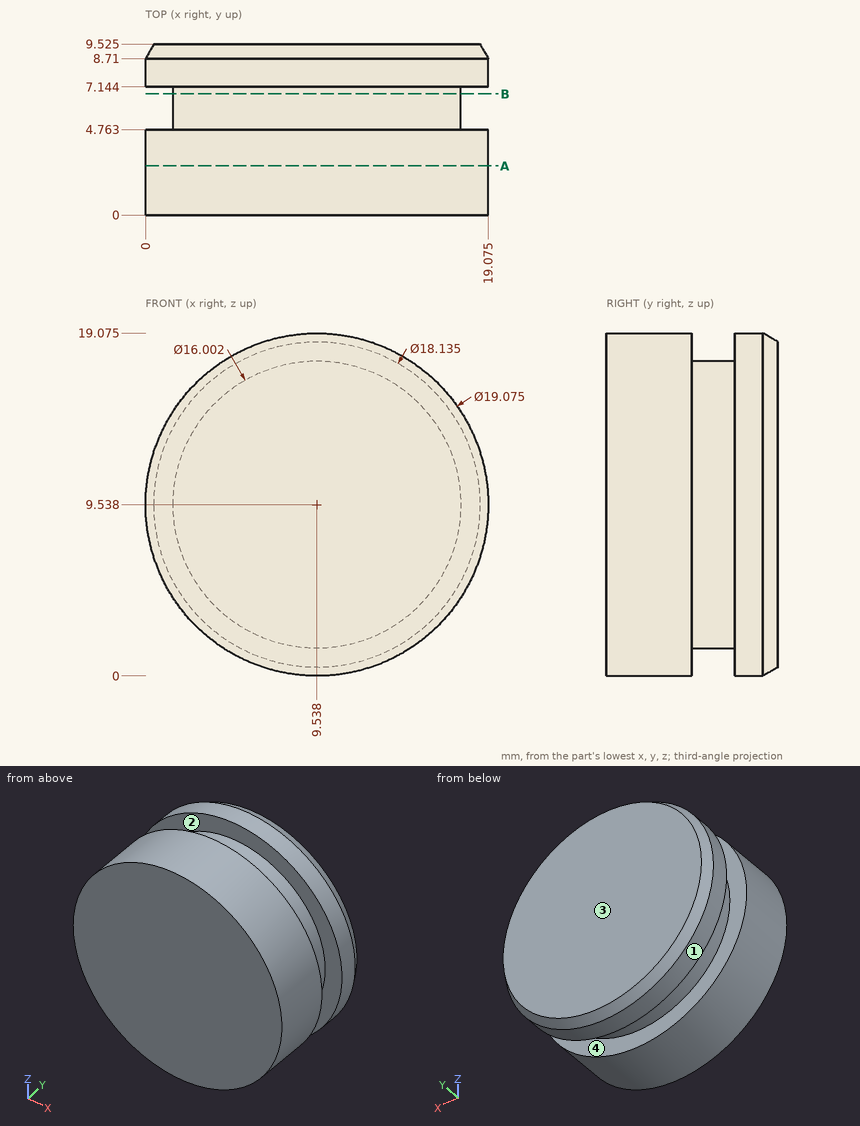
Input: dimensioned drawing with shaded views. Units: mm. Origin: part minimum x, y, z. Round coordinates to 2 decimals unless told otherwise and drop trailing zeros. Loops run counter-clockwise (first coordinate to the right, second up) from the corner with the lowest first, then second, coordinate; pieces in that order, holes last. Notation, with made-up numbers: M -39.75,72.25 L 12.25,72.25 A12 cw 12.25,84.25 Z; hole C 54,-18 d10. An arc over 180 degrees is marked long. Answer in a Markdown table with one row per item. Add a question column.
1. Mould query, pull axis Y, two halves, no side actions, for the marked faces 1, 2, 3 and 4. Classes: released by +Y, released by -Y, zero draft, split by the parting line, or undercut.
2. Contact query for flat-ended pins moving along their axis: pin 1 (2 mm diameter, centred on x = 13.5, y = 5.5, fed in from +Z); pin 2 (5 mm diameter, centred on x = 2.5, y = 6.5, fed in from +Z); pin 3 (4 mm diameter, centred on y = 3, z = 15.5, fed in from -X). Output: stop coordinate, or through.
3. Ray query, probe 1 along Z at (x, y) = (1, 1.5) (1 decimal); probe 2 along Z at (x, y) = (11.75, 4.5) (1 decimal); probe 3 along X at (y, z) = (2.5, 4.75) (1 decimal). Return the intervals inside material, ascending.
4. Section B-B (y = 6.75). Output: boundary loops of the cut face in (x, z), and give its area (3 significant figures).
5. Section A-A (y = 2.75). Output: boundary loops of the cut face in (x, z) (1 decimal), and give its area (3 significant figures).
Values follow:
| question | item | result |
|---|---|---|
| 1 | face 1 | zero draft |
| 1 | face 2 | undercut |
| 1 | face 3 | released by +Y |
| 1 | face 4 | undercut |
| 2 | pin 1 | z = 18.49 |
| 2 | pin 2 | z = 17.88 |
| 2 | pin 3 | x = 0.86 |
| 3 | probe 1 | 5.3 to 13.8 |
| 3 | probe 2 | 0.3 to 18.8 |
| 3 | probe 3 | 1.3 to 17.8 |
| 4 | outline | C 9.54,9.54 d16 |
| 4 | area | 201 mm^2 |
| 5 | outline | C 9.5,9.5 d19.1 |
| 5 | area | 286 mm^2 |
